CAD build for the part. Positions are in the model's coordinates, mm. A direction names the side the tool comes from. Give positions to 0.01 mm unless a question says otherwise; leave off trailing zeros. Loops run counter-clockwise (first coordinate to the right, second up) from the corner with the lowest first, then second, coordinate; pieces in that order, holes last. Notation, with made-up numbers: M -38,72.25 L -17,72.25 A35 cw -17,104.25 Z; hole C 6,-40 d6. An arc over 180 degrees is marked long. One line per question, with ' | ' between items.
```python
from build123d import *

# Parameters (mm, degrees)
SKETCH_2_W      = 53
SKETCH_2_H      = 23
EXTRUDE_1_DEPTH = 19
SKETCH_3_R      = 2.5
EXTRUDE_2_DEPTH = 9
EXTRUDE_START   = 9
SKETCH_7_R      = 2.5
EXTRUDE_5_DEPTH = 9


with BuildPart() as part:
    # 草图2 → 凸台-拉伸1 (new body)
    with BuildSketch(Plane(origin=(0, 0, 0), x_dir=(0, 0, -1), z_dir=(1, 0, 0))):
        with Locations((-9.248715633, 27.370444178)):
            Rectangle(SKETCH_2_W, SKETCH_2_H)
    extrude(amount=EXTRUDE_1_DEPTH)

    # 草图3 → 凸台-拉伸2 (add)
    with BuildSketch(Plane(origin=(19, 0, 0), x_dir=(0, 0, -1), z_dir=(1, 0, 0))):
        with Locations(Location((6.251284367, 27.370444178, 0), (0, 0, 180))):
            Circle(SKETCH_3_R)
    extrude(amount=EXTRUDE_2_DEPTH)

    # 草图7 → 凸台-拉伸5 (add)
    with BuildSketch(Plane.ZY.offset(EXTRUDE_START)):
        with Locations((-6.251284367, 27.370444178)):
            Circle(SKETCH_7_R)
    extrude(amount=-EXTRUDE_5_DEPTH)


solid = part.part
```
Item 1: Drop flat-ended pins along their axis: P1, Ø11.5, axis at y = 29, z = 7, coming from the -X side; P2, Ø4, axis at y = 25.5, z = 13.5, coming from the +X side; P3, Ø1, axis at x = -1, z = 1.5, coming from the +Y side. Give the stop position or say it passes through.
Conclusion:
P1: x = 0 | P2: x = 19 | P3: through
Item 2: Saw through at D-D on y = 26.25. Give the cut face in (x, z), and give its area (3 significant figures).
Conclusion:
outline: M -9,-8.49 L 0,-8.49 L 0,-17.25 L 19,-17.25 L 19,-8.49 L 28,-8.49 L 28,-4.02 L 19,-4.02 L 19,35.75 L 0,35.75 L 0,-4.02 L -9,-4.02 Z | area: 1,090 mm²
Item 3: Drill centre line: line 1 along X through (y, z) = (25, 26). Where is it in solid material? Low to high. Write a range as [from, to].
Conclusion:
line 1: [0, 19]
Item 4: 3-axis set-ups, long thin cutter, end or side, ignore diameter. For faces 1 (the cylindrical face through (23.437, 24.892, -6.577)), 2 (the flat face through (9, 27, -17.251)), 3 (the cylindrical face through (-4.56, 29.85, -6.58)): which of +Z, -Z, +X, -X, +Y, -Y reach the whole face in a straight line?
Conclusion:
face 1: +X | face 2: -Z, +X, -X, +Y, -Y | face 3: -X
Item 5: Saw through at C-C on x = 25.5. Give the cut face in (y, z).
Conclusion:
outline: C 27.37,-6.25 d5
Item 6: Saw through at B-B on z = 8.5. Give the cut face in (x, y).
Conclusion:
outline: M 0,15.87 L 19,15.87 L 19,38.87 L 0,38.87 Z
Item 7: Saw through at A-A on y = 30.5. Give the cut face in (x, z), and give its area (3 significant figures).
Conclusion:
outline: M 0,-17.25 L 19,-17.25 L 19,35.75 L 0,35.75 Z | area: 1,010 mm²
